from build123d import *

# Parameters (mm, degrees)
SKETCH2_W                  = 127
SKETCH2_H                  = 736.6
BOSS_EXTRUDE1_DEPTH        = 25.4
F_1_2_0_5_DIAMETER_HOLE1_D = 50.8
F_1_2_0_5_DIAMETER_HOLE2_D = 12.7
FILLET1_R                  = 25.4


with BuildPart() as part:
    # Sketch2 → Boss-Extrude1 (new body)
    with BuildSketch(Plane(origin=(0, 0, 0), x_dir=(1, 0, 0), z_dir=(0, 1, 0))):
        with Locations((-63.5, 368.3)):
            Rectangle(SKETCH2_W, SKETCH2_H)
    extrude(amount=BOSS_EXTRUDE1_DEPTH)

    # 1/2 (0.5) Diameter Hole1 (through all)
    with Locations(Plane(origin=(0, 25.4, 0), x_dir=(1, 0, 0), z_dir=(0, 1, 0))):
        with Locations((-63.5, 673.1), (-63.5, 63.5)):
            Hole(F_1_2_0_5_DIAMETER_HOLE1_D / 2)

    # 1/2 (0.5) Diameter Hole2 (through all)
    with Locations(Plane(origin=(0, 25.4, 0), x_dir=(1, 0, 0), z_dir=(0, 1, 0))):
        with Locations((-93.923508124, 703.915980712), (-33.076491876, 703.915980712), (-33.076491876, 642.284019288), (-93.923508124, 642.284019288), (-63.5, 602.937236364), (-63.5, 552.137236364), (-63.5, 501.337236364), (-63.5, 450.537236364), (-63.5, 399.737236364), (-63.5, 348.937236364), (-63.5, 298.137236364), (-63.5, 247.337236364), (-63.5, 196.537236364), (-93.923508124, 32.684019288), (-93.923508124, 94.315980712), (-33.076491876, 94.315980712), (-33.076491876, 32.684019288)):
            Hole(F_1_2_0_5_DIAMETER_HOLE2_D / 2)

    # Fillet1
    fillet1_edges = [part.edges().sort_by_distance(p)[0] for p in [
        (0, 12.7, 0),
        (-127, 12.7, 0),
        (-127, 12.7, -736.6),
        (0, 12.7, -736.6),
    ]]
    fillet(fillet1_edges, radius=FILLET1_R)


solid = part.part
Read the model definition and answer for the solid it produces. Units are mm, in the model's axes. Give positions to 0.01 mm unless a question says otherwise; leave off trailing zeros. Write each loop counter-clockwise with the first axis right and the second up, starting at its lowest first coordinate (ties: lowest second). Pieces come first, ordered by that corner, then holes. Notation, with made-up numbers: (20, 76) - (69, 76) arc R23 ccw to (69, 91) - close; hole circle Ø11 at (-4, -35). An arc over 180 degrees is marked (long way). Return JSON: item names as keys, results as strings.
Q1. A cutting plane is placed at A-A, the plane z = -63.5. Determine the outline of the cut face in (x, y).
Reply:
{"outline": "(-127, 0) - (-88.9, 0) - (-88.9, 25.4) - (-127, 25.4) - close; (-38.1, 0) - (0, 0) - (0, 25.4) - (-38.1, 25.4) - close"}
Q2. A cutting plane is placed at D-D, the plane x = -118. Determine the outline of the cut face in (y, z), and give its area (3 significant figures).
Reply:
{"outline": "(0, -730.6) - (25.4, -730.6) - (25.4, -6) - (0, -6) - close", "area": "18,400 mm²"}
Q3. A cutting plane is placed at B-B, the plane y = 4. Count the separate pieces of the cut face and the enclosed holes in it, and give its area (3 significant figures).
Reply:
{"separate pieces": "1", "enclosed holes": "19", "area": "86,800 mm²"}
Q4. For a pull along X with two mould halves and no side action, classify faces 1 (the face through (0, 13, -363)), 2 (the face through (-36.01, 12.52, -27.05)), 3 (the face through (-64, 13, 0)) as released by +X, released by -X, zero draft, split by the parting line, or undercut.
Reply:
{"face 1": "released by +X", "face 2": "undercut", "face 3": "zero draft"}
Q5. Given P1, Ø2, axis at x = -13, y = 14, coming from the +Z side, flat-ended and moving along its own axis, determine where the tip first touches the part or whether it passes through.
Reply:
{"P1": "z = -2.7"}
Q6. Consider line 1 along Z through (x, y) = (-93, 11.75); line 2 along Z through (x, y) = (-33, 14.5); line 3 along Z through (x, y) = (-42, 20.75). Determine where each line is inside the solid, lowest interval first. Write a range as [from, to].
Reply:
{"line 1": "[-736.6, -710.2], [-697.63, -648.57], [-636, -100.6], [-88.03, -38.97], [-26.4, 0]", "line 2": "[-736.6, -710.27], [-697.57, -648.63], [-635.93, -100.67], [-87.97, -39.03], [-26.33, 0]", "line 3": "[-736.6, -686.62], [-659.58, -77.02], [-49.98, 0]"}
